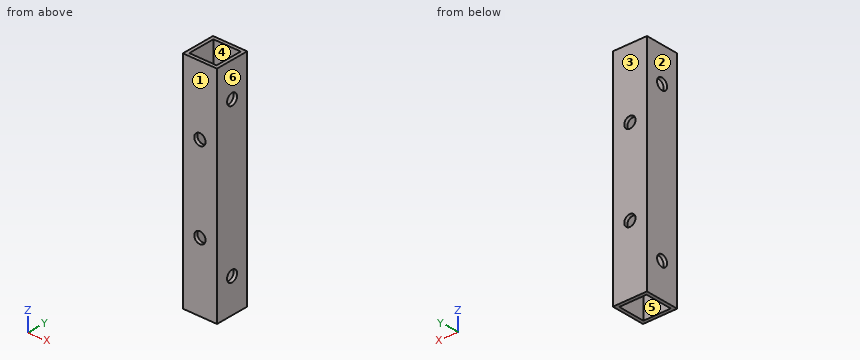
Autodesk Inventor part; units mm, degrees
ref_plane "YZ Plane" through (0, 0, 0) normal (1, 0, 0) x (0, 1, 0)
ref_plane "XZ Plane" through (0, 0, 0) normal (0, 1, 0) x (-1, 0, 0)
ref_plane "XY Plane" through (0, 0, 0) normal (0, 0, 1) x (1, 0, 0)
sketch "スケッチ1" plane through (0, 0, 0) normal (0, 0, 1) x (1, 0, 0)
  line L0 (5, -5) -> (-5, -5)
  line L1 (-5, -5) -> (-5, 5)
  line L2 (-5, 5) -> (5, 5)
  line L3 (5, 5) -> (5, -5)
  line L4 (5, -5) -> (-5, 5) construction
  line L5 (-5, -5) -> (5, 5) construction
  line L6 (4, 4) -> (-4, 4)
  line L7 (-4, 4) -> (-4, -4)
  line L8 (-4, -4) -> (4, -4)
  line L9 (4, -4) -> (4, 4)
  point P0 (0, 0)
  dimension "d0" = 10
  dimension "d1" = 10
  dimension "d2" = 1
extrude "押し出し1" add sketch "スケッチ1" along normal blind 65
sketch "スケッチ2" plane through (5, -5, 0) normal (1, 0, 0) x (0, 0, -1)
  line L0 (0, 5) -> (-65, 5)
  line L1 (-65, 9) -> (-65, 1)
  line L2 (0, 0) -> (0, 10)
  point P0 (-55, 5)
  point P1 (-10, 5)
  dimension "d5" = 45
  dimension "d6" = 10
hole "穴1" at (5, 0, 55) at (5, 0, 10) direction (-1, 0, 0) diameter 3.3 end through all
sketch "スケッチ3" plane through (-5, 5, 0) normal (0, 1, 0) x (1, 0, 0)
  line L0 (5, 0) -> (5, -65)
  line L1 (1, -65) -> (9, -65)
  line L2 (10, 0) -> (0, 0)
  point P0 (5, -45)
  point P1 (5, -20)
  dimension "d14" = 20
  dimension "d15" = 25
hole "穴2" at (0, 5, 45) at (0, 5, 20) direction (0, -1, 0) diameter 3.3 end through all
properties part number "xxkaku_1010"
Can you work these out from the model? Positions are in its coordinate system, mm. Face numbers are marked on the shaded views. A direction names the side the tool comes from. Coordinates: 2 decimals unless noted, no trailing zeros. Loops run counter-clockwise (first coordinate to the right, second up) from the corner with the lowest first, then second, coordinate; pieces in that order, holes last.
1) Thinking about a two-plate mould opening in Y: for the marked faces 1, 2, 3 and 4, which applies, pulls with the +Y half, pulls with the -Y half, needs draft (parallel to the pull), parting line crosses it, or undercut?
2) Imagine slicing it at D-D on z = 13.5. List the corners of the cut face in (x, y) for me, plus the area to 3 significant figures.
3) Which directions (+Z, -Z, +X, -X, +Y, -Y) give clear straight access to the entire face, cutting with the end or side of a thin tool? Please do the marked faces 5 and 6.
4) Imagine slicing it at A-A on x = 0. List the corners of the cut face in (y, z) for me.
5) I need wall thicknesses on probe 1 along X at (y, z) = (-0.75, 30.5); probe 2 along X at (y, z) = (-4.5, 20). Which ranges of each line are inside material? Lowest first, please.
6) Imagine slicing it at B-B on z = 45. List the corners of the cut face in (x, y) for me.
7) For pin 1 (4 mm diameter, centred on x = 1, y = -0.5, fed in from -Z), with a flat end and sliding along its axis, tell me the tip position at first contact or that it passes through.
8) Imagine slicing it at C-C on y = -3. List the corners of the cut face in (x, z) for me, plus the area to 3 significant figures.
Completed:
1. face 1: pulls with the -Y half
1. face 2: needs draft
1. face 3: pulls with the +Y half
1. face 4: undercut
2. outline: (-5, -5) - (5, -5) - (5, 5) - (-5, 5) - close; hole (-4, -4) - (4, -4) - (4, 4) - (-4, 4) - close
2. area: 36.0 mm2
3. face 5: +Z, -Z
3. face 6: +Z, -Z, +X, +Y, -Y
4. outline: (-5, 0) - (-4, 0) - (-4, 18.35) - (-5, 18.35) - close; (-5, 21.65) - (-4, 21.65) - (-4, 43.35) - (-5, 43.35) - close; (-5, 46.65) - (-4, 46.65) - (-4, 65) - (-5, 65) - close; (4, 0) - (5, 0) - (5, 18.35) - (4, 18.35) - close; (4, 21.65) - (5, 21.65) - (5, 43.35) - (4, 43.35) - close; (4, 46.65) - (5, 46.65) - (5, 65) - (4, 65) - close
5. probe 1: x = -5 to -4, 4 to 5
5. probe 2: x = -5 to -1.65, 1.65 to 5
6. outline: (-5, -5) - (-1.65, -5) - (-1.65, -4) - (-4, -4) - (-4, 4) - (-1.65, 4) - (-1.65, 5) - (-5, 5) - close; (1.65, -5) - (5, -5) - (5, 5) - (1.65, 5) - (1.65, 4) - (4, 4) - (4, -4) - (1.65, -4) - close
7. pin 1: passes through
8. outline: (-5, 0) - (-4, 0) - (-4, 65) - (-5, 65) - close; (4, 0) - (5, 0) - (5, 65) - (4, 65) - close
8. area: 130 mm2
